Model file for the job. Use its own axes, mm. A direction names the side the tool comes from. Round coordinates to 2 decimals unless told otherwise and drop trailing zeros. Order: outer loops, then holes, each group sorted by start corner. A loop starts at its lowest first (then second) coordinate and runs counter-clockwise, first axis right, second up. Notation, with made-up numbers: (-1.5, 33.5) - (48.5, 33.5) arc R17 ccw to (48.5, 60.5) - close; hole circle Ø7 at (-23, 62.25). An arc over 180 degrees is marked (long way). Write item = value, one per line.
```python
from build123d import *

# Parameters (mm, degrees)
F1_DEPTH = 3


with BuildPart() as f1:
    # F0 (on Top) → F1 (new body)
    with BuildSketch(Plane.XY):
        with BuildLine():
            ThreePointArc((97.5, 0), (89.426248, 16.792435), (71.268757, 20.972967))
            ThreePointArc((71.268757, 20.972967), (42.645894, 19.743038), (15.405524, 28.616775))
            ThreePointArc((15.405524, 28.616775), (-16.666891, 27.900981), (-32.5, 0))
            ThreePointArc((-32.5, 0), (-16.666891, -27.900981), (15.405524, -28.616775))
            ThreePointArc((15.405524, -28.616775), (42.645894, -19.743038), (71.268757, -20.972967))
            ThreePointArc((71.268757, -20.972967), (89.426248, -16.792435), (97.5, 0))
        make_face()
        with BuildLine():
            ThreePointArc((13.035443, 24.214195), (41.968056, 14.789198), (72.369046, 16.095533))
            ThreePointArc((72.369046, 16.095533), (86.303865, 12.887217), (92.5, 0))
            ThreePointArc((92.5, 0), (86.303865, -12.887217), (72.369046, -16.095533))
            ThreePointArc((72.369046, -16.095533), (41.968056, -14.789198), (13.035443, -24.214195))
            ThreePointArc((13.035443, -24.214195), (-14.102754, -23.608523), (-27.5, 0))
            ThreePointArc((-27.5, 0), (-14.102754, 23.608523), (13.035443, 24.214195))
        make_face(mode=Mode.SUBTRACT)
    extrude(amount=F1_DEPTH)


solid = f1.part
```
1) Mould opens along X. For faces 1 (the face through (32, 17, 3)), 2 (the face through (41.54, 14.85, 1.48)) say: +X half, -X half, draft (parallel to the pull), parting line (faces both ways), or undercut.
Conclusion:
face_1 = draft
face_2 = undercut
2) Cut at B-B (y = 11). Write the cut outline in (x, z), and give its area (3 significant figures).
Conclusion:
outline = (-30.58, 0) - (-25.2, 0) - (-25.2, 3) - (-30.58, 3) - close; (88.3, 0) - (94.47, 0) - (94.47, 3) - (88.3, 3) - close
area = 34.7 mm^2
3) Cut at A-A (x = 89). Write the cut outline in (y, z), and give its area (3 significant figures).
Conclusion:
outline = (-17.12, 0) - (-10.16, 0) - (-10.16, 3) - (-17.12, 3) - close; (10.16, 0) - (17.12, 0) - (17.12, 3) - (10.16, 3) - close
area = 41.8 mm^2
4) Wall check: line 1 along X through (y, z) = (0.5, 1.1); line 2 along Y through (x, z) = (75.5, 0.35); line 3 along Y through (x, z) = (-17, 2.25). Give the ranges that are in metal, low to high.
Conclusion:
line_1 = -32.5 to -27.5, 92.49 to 97.49
line_2 = -21.49 to -16.49, 16.49 to 21.49
line_3 = -27.7 to -21.62, 21.62 to 27.7
5) 3-axis set-ups, long thin cutter, end or side, ignore diameter. For faces 3 (the face through (42.393, -14.732, 1.479)), 4 (the face through (32, 17, 0)): which of +Z, -Z, +X, -X, +Y, -Y reach the whole face in a straight line?
Conclusion:
face_3 = +Z, -Z
face_4 = -Z, +X, -X, +Y, -Y
6) Cut at C-C (z = 0.85). Write the cut outline in (x, y).
Conclusion:
outline = (15.41, -28.62) arc R80.49 cw to (71.27, -20.97) arc R21.5 ccw (long way) to (71.27, 20.97) arc R80.49 cw to (15.41, 28.62) arc R32.5 ccw (long way) to start; hole (-27.5, 0) arc R27.5 ccw to (13.04, -24.21) arc R85.49 cw to (72.37, -16.1) arc R16.5 ccw (long way) to (72.37, 16.1) arc R85.49 cw to (13.04, 24.21) arc R27.5 ccw to start
7) Flat gauge pin, fed straight in: pin 1 Ø1.5 at (y, z) = (-7, 1) entering from -X. Where does the tip first touch, or does it go through?
Conclusion:
pin_1 = -31.89
